from build123d import *

# Parameters (mm, degrees)
F1_DEPTH = 3.1
F2_DEPTH = 3.1


# Not quite as in the source:
# - a feature names something its author has since deleted; it is built from what else it names


with BuildPart() as f1:
    # F0 (on Top) → F1 (new body)
    with BuildSketch(Plane.XY):
        with BuildLine():
            ThreePointArc((-38.8921249823, 64.9047296424), (-32.2549034273, 66.6273143387), (-28.3365694268, 61))
            ThreePointArc((-28.3365694268, 61), (-32.2549034273, 55.3726856613), (-38.8921249823, 57.0952703576))
            ThreePointArc((-38.8921249823, 57.0952703576), (-40.607834636, 53.3556046539), (-43.3365694268, 50.2761947052))
            ThreePointArc((-43.3365694268, 50.2761947052), (-39.1254485166, 47.8445206449), (-34.3365694268, 47))
            ThreePointArc((-34.3365694268, 47), (-24.4370744902, 51.1005050634), (-20.3365694268, 61))
            ThreePointArc((-20.3365694268, 61), (-24.4370744902, 70.8994949366), (-34.3365694268, 75))
            ThreePointArc((-34.3365694268, 75), (-39.1254485166, 74.1554793551), (-43.3365694268, 71.7238052948))
            ThreePointArc((-43.3365694268, 71.7238052948), (-40.607834636, 68.6443953461), (-38.8921249823, 64.9047296424))
        make_face()
        with BuildLine():
            ThreePointArc((-52.3365694268, 75), (-47.547690337, 74.1554793551), (-43.3365694268, 71.7238052948))
            ThreePointArc((-43.3365694268, 71.7238052948), (-39.1254485166, 74.1554793551), (-34.3365694268, 75))
            Line((-34.3365694268, 75), (-52.3365694268, 75))
        make_face()
        with BuildLine():
            ThreePointArc((-47.6959444268, 65.1865379025), (-45.9842893254, 68.7672788776), (-43.3365694268, 71.7238052948))
            ThreePointArc((-43.3365694268, 71.7238052948), (-47.547690337, 74.1554793551), (-52.3365694268, 75))
            ThreePointArc((-52.3365694268, 75), (-66.3365694268, 61), (-52.3365694268, 47))
            ThreePointArc((-52.3365694268, 47), (-47.547690337, 47.8445206449), (-43.3365694268, 50.2761947052))
            ThreePointArc((-43.3365694268, 50.2761947052), (-45.9842893254, 53.2327211224), (-47.6959444268, 56.8134620975))
            ThreePointArc((-47.6959444268, 56.8134620975), (-58.5865694268, 61), (-47.6959444268, 65.1865379025))
        make_face()
        with BuildLine():
            ThreePointArc((-34.3365694268, 47), (-39.1254485166, 47.8445206449), (-43.3365694268, 50.2761947052))
            ThreePointArc((-43.3365694268, 50.2761947052), (-47.547690337, 47.8445206449), (-52.3365694268, 47))
            Line((-52.3365694268, 47), (-34.3365694268, 47))
        make_face()
        with BuildLine():
            ThreePointArc((-40.3365694268, 61), (-39.9638837655, 63.0816659995), (-38.8921249823, 64.9047296424))
            ThreePointArc((-38.8921249823, 64.9047296424), (-40.607834636, 68.6443953461), (-43.3365694268, 71.7238052948))
            ThreePointArc((-43.3365694268, 71.7238052948), (-45.9842893254, 68.7672788776), (-47.6959444268, 65.1865379025))
            ThreePointArc((-47.6959444268, 65.1865379025), (-46.5027710822, 63.2426093898), (-46.0865694268, 61))
            Line((-46.0865694268, 61), (-40.3365694268, 61))
        make_face()
        with BuildLine():
            ThreePointArc((-43.3365694268, 50.2761947052), (-40.607834636, 53.3556046539), (-38.8921249823, 57.0952703576))
            ThreePointArc((-38.8921249823, 57.0952703576), (-39.9638837655, 58.9183340005), (-40.3365694268, 61))
            Line((-40.3365694268, 61), (-46.0865694268, 61))
            ThreePointArc((-46.0865694268, 61), (-46.5027710822, 58.7573906102), (-47.6959444268, 56.8134620975))
            ThreePointArc((-47.6959444268, 56.8134620975), (-45.9842893254, 53.2327211224), (-43.3365694268, 50.2761947052))
        make_face()
    extrude(amount=F1_DEPTH)

    # F0 (on Top) → F2 (join)
    with BuildSketch(Plane.XY):
        with BuildLine():
            ThreePointArc((-38.8921249823, 64.9047296424), (-32.2549034273, 66.6273143387), (-28.3365694268, 61))
            ThreePointArc((-28.3365694268, 61), (-32.2549034273, 55.3726856613), (-38.8921249823, 57.0952703576))
            ThreePointArc((-38.8921249823, 57.0952703576), (-40.607834636, 53.3556046539), (-43.3365694268, 50.2761947052))
            ThreePointArc((-43.3365694268, 50.2761947052), (-39.1254485166, 47.8445206449), (-34.3365694268, 47))
            ThreePointArc((-34.3365694268, 47), (-24.4370744902, 51.1005050634), (-20.3365694268, 61))
            ThreePointArc((-20.3365694268, 61), (-24.4370744902, 70.8994949366), (-34.3365694268, 75))
            ThreePointArc((-34.3365694268, 75), (-39.1254485166, 74.1554793551), (-43.3365694268, 71.7238052948))
            ThreePointArc((-43.3365694268, 71.7238052948), (-40.607834636, 68.6443953461), (-38.8921249823, 64.9047296424))
        make_face()
        with BuildLine():
            ThreePointArc((-52.3365694268, 75), (-47.547690337, 74.1554793551), (-43.3365694268, 71.7238052948))
            ThreePointArc((-43.3365694268, 71.7238052948), (-39.1254485166, 74.1554793551), (-34.3365694268, 75))
            Line((-34.3365694268, 75), (-52.3365694268, 75))
        make_face()
        with BuildLine():
            ThreePointArc((-47.6959444268, 65.1865379025), (-45.9842893254, 68.7672788776), (-43.3365694268, 71.7238052948))
            ThreePointArc((-43.3365694268, 71.7238052948), (-47.547690337, 74.1554793551), (-52.3365694268, 75))
            ThreePointArc((-52.3365694268, 75), (-66.3365694268, 61), (-52.3365694268, 47))
            ThreePointArc((-52.3365694268, 47), (-47.547690337, 47.8445206449), (-43.3365694268, 50.2761947052))
            ThreePointArc((-43.3365694268, 50.2761947052), (-45.9842893254, 53.2327211224), (-47.6959444268, 56.8134620975))
            ThreePointArc((-47.6959444268, 56.8134620975), (-58.5865694268, 61), (-47.6959444268, 65.1865379025))
        make_face()
        with BuildLine():
            ThreePointArc((-34.3365694268, 47), (-39.1254485166, 47.8445206449), (-43.3365694268, 50.2761947052))
            ThreePointArc((-43.3365694268, 50.2761947052), (-47.547690337, 47.8445206449), (-52.3365694268, 47))
            Line((-52.3365694268, 47), (-34.3365694268, 47))
        make_face()
    extrude(amount=F2_DEPTH)


solid = f1.part
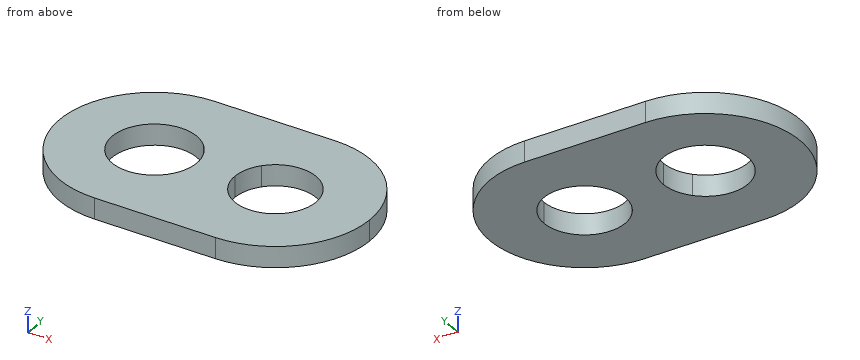
CAD build for the part. Positions are in the model's coordinates, mm. Round coordinates to 2 decimals unless told otherwise and drop trailing zeros. Loops run counter-clockwise (first coordinate to the right, second up) from the corner with the lowest first, then second, coordinate; pieces in that order, holes last. Notation, with made-up numbers: (-16.75, 68.25) - (13.25, 68.25) arc R18 ccw to (13.25, 97.25) - close; hole circle Ø1 at (16.25, 50.25). An arc over 180 degrees is marked (long way). Put each result on its own line as item: value.
1. Slice it at A-A on z = 2.65. List the corners of the cut face in (x, y).
Geometry check:
outline: (-52.34, 47) - (-34.34, 47) arc R14 ccw to (-34.34, 75) - (-52.34, 75) arc R14 ccw to start; hole circle Ø12.5 at (-52.34, 61); hole circle Ø12 at (-34.34, 61)
2. Slice it at B-B on y = 63.5. List the corners of the cut face in (x, z), and give its area (3 significant figures).
Geometry check:
outline: (-66.11, 0) - (-58.06, 0) - (-58.06, 3.1) - (-66.11, 3.1) - close; (-46.61, 0) - (-39.79, 0) - (-39.79, 3.1) - (-46.61, 3.1) - close; (-28.88, 0) - (-20.56, 0) - (-20.56, 3.1) - (-28.88, 3.1) - close
area: 71.9 mm²
3. Wall check: line 1 (X direction, y = 61, z = 2.2); line 2 (Y direction, x = -52, z = 2); line 3 (X direction, y = 62.25, z = 2.3). Give the ranges that are in metal, low to high.
Geometry check:
line 1: -66.34 to -58.59, -46.09 to -40.34, -28.34 to -20.34
line 2: 47 to 54.76, 67.24 to 75
line 3: -66.28 to -58.46, -46.21 to -40.2, -28.47 to -20.39
4. Slice it at D-D on y = 55.5. List the corners of the cut face in (x, z).
Geometry check:
outline: (-65.21, 0) - (-55.31, 0) - (-55.31, 3.1) - (-65.21, 3.1) - close; (-49.37, 0) - (-36.73, 0) - (-36.73, 3.1) - (-49.37, 3.1) - close; (-31.94, 0) - (-21.46, 0) - (-21.46, 3.1) - (-31.94, 3.1) - close
5. Slice it at C-C on x = -58. List the corners of the cut face in (y, z), and give its area (3 significant figures).
Geometry check:
outline: (48.2, 0) - (58.36, 0) - (58.36, 3.1) - (48.2, 3.1) - close; (63.64, 0) - (73.8, 0) - (73.8, 3.1) - (63.64, 3.1) - close
area: 63.0 mm²
6. Pin check, flat tips, straight feed: P1, Ø1, axis at y = 64, z = 2, coming from the -X side; P2, Ø1.5, axis at y = 71, z = 2.5, coming from the -X side. Stop position of each tip, or through.
Geometry check:
P1: x = -66.11
P2: x = -62.85
